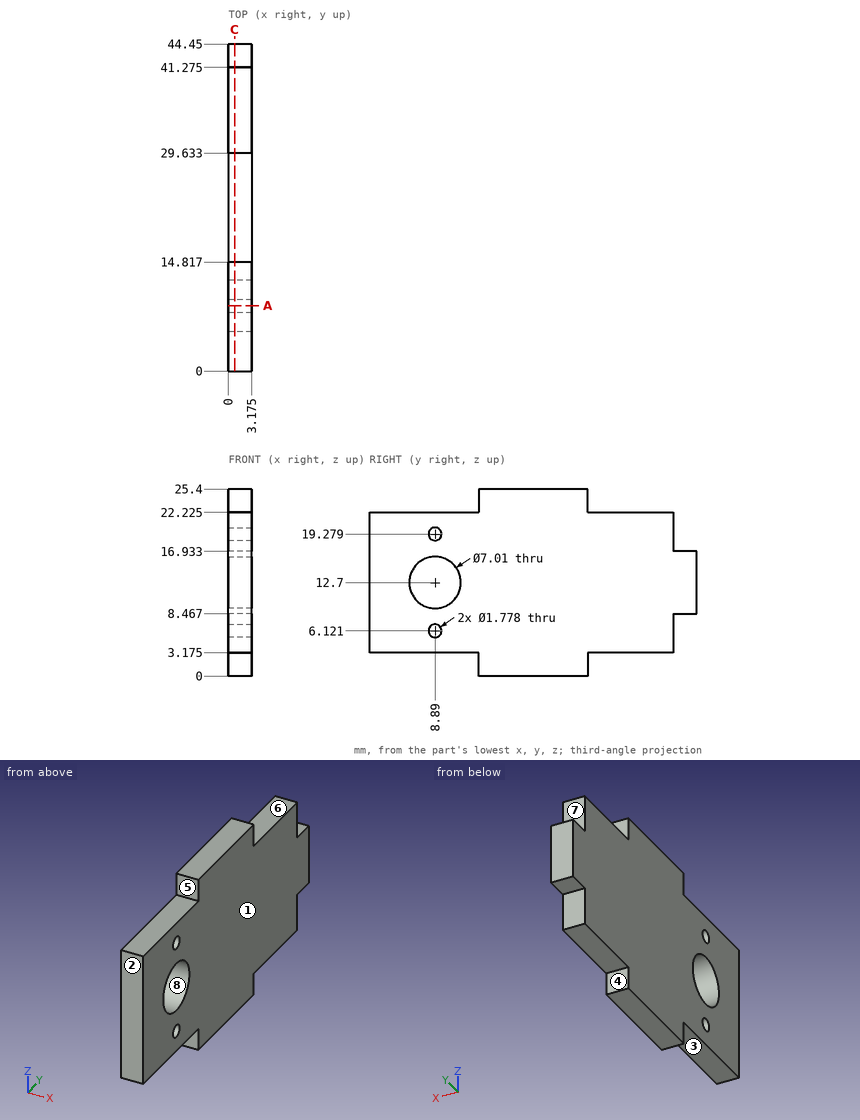
Geometry check sheet. Reference: drawing and pictorial views, mm from the part's lowest x, y, z. A direction names the side the tool comes from. Round coordinates to 2 decimals unless told otherwise and drop trailing zeros. Order: outer loops, then holes, each group sorted by start corner. A loop starts at its lowest first (then second) coordinate and runs counter-clockwise, first axis right, second up.
Q1. Draft check along Y on the marked faces 6, 7 and 8. Enter one of: pulls with the +Y half, pulls with the -Y half, needs draft (parallel to the pull), parting line crosses it, or undercut.
Filled sheet:
face 6: needs draft
face 7: pulls with the +Y half
face 8: undercut
Q2. Cross-section at A-A, the plane y = 8.89. Enter the section's corners in (x, z) (1 decimal).
Filled sheet:
outline: (0, 3.2) - (3.2, 3.2) - (3.2, 5.2) - (0, 5.2) - close; (0, 7) - (3.2, 7) - (3.2, 9.2) - (0, 9.2) - close; (0, 16.2) - (3.2, 16.2) - (3.2, 18.4) - (0, 18.4) - close; (0, 20.2) - (3.2, 20.2) - (3.2, 22.2) - (0, 22.2) - close
Q3. Scan lines: L1, parallel to Z at x = 1, y = 9 (1 decimal); L2, parallel to Y at x = 0.2, z = 6 (1 decimal); L3, parallel to Y at x = 2.65, z = 17.25 (1 decimal). Record each from-to range of solid material in increasing order.
Filled sheet:
L1: z = 3.2 to 5.2, 7 to 9.2, 16.2 to 18.4, 20.2 to 22.2
L2: y = 0 to 8, 9.8 to 41.3
L3: y = 0 to 41.3
Q4. Set-up check for the marked faces 1, 2, 3, 4 and 5: record each of +Z, -Z, +X, -X, +Y, -Y from which the full face is reachable in a straight line by a thin tool's end or side.
Filled sheet:
face 1: +Z, -Z, +X, +Y, -Y
face 2: +Z, -Z, +X, -X, -Y
face 3: -Z, +X, -X, -Y
face 4: -Z, +X, -X, +Y
face 5: +Z, +X, -X, -Y
Q5. Depth check by flat-ended pin: P1, Ø1, axis at x = 2, y = 42.5, coming from the +Z side; P2, Ø1, axis at x = 1, z = 24, coming from the -Y side; P3, Ø1, axis at x = 2, y = 33, coming from the +Z side (3 decimals). Enter the tip coordinate at first touch or a pass-through.
Filled sheet:
P1: stops at z = 16.93
P2: stops at y = 14.82
P3: stops at z = 22.225
Q6. Cross-section at C-C, the plane x = 0.85. Give the number of separate pieces and of enclosed holes in the cut face, plus the area to 3 significant figures.
Filled sheet:
separate pieces: 1
enclosed holes: 3
area: 864 mm2
